Build history of the part. All positions in model axes, mm. A direction names the side the tool comes from. Coordinates: 2 decimals unless noted, no trailing zeros. Order: outer loops, then holes, each group sorted by start corner. A loop starts at its lowest first (then second) coordinate and runs counter-clockwise, first axis right, second up. Notation, with made-up numbers: M 41.25,18.5 L 74.25,18.5 A12 ccw 74.25,24.5 Z; hole C 88,-38 d11. An arc over 180 degrees is marked long. Use a Markdown table: item, result. Add a question column.
from build123d import *

# Parameters (mm, degrees)
SKETCH1_R                     = 8
BOSS_EXTRUDE1_DEPTH           = 1.6
SKETCH2_R                     = 6.07
BOSS_EXTRUDE2_DEPTH           = 8.2
BOSS_EXTRUDE3_START           = -1.6
SKETCH3_R                     = 8
BOSS_EXTRUDE3_DEPTH           = 1.6
SKETCH4_R                     = 6.35
BOSS_EXTRUDE4_DEPTH           = 5.6
F_5_0_5_DIAMETER_HOLE1_D      = 5
F_3_0_3_DIAMETER_HOLE1_REACH  = 23.882
F_3_0_3_DIAMETER_HOLE1_BORE_R = 1.5


with BuildPart() as part:
    # Sketch1 → Boss-Extrude1 (new body)
    with BuildSketch(Plane.XY.offset(1.6)):
        with Locations(Location((0, 0, 0), (0, 0, 180))):
            Circle(SKETCH1_R)
    extrude(amount=-BOSS_EXTRUDE1_DEPTH)

    # Sketch2 → Boss-Extrude2 (add)
    with BuildSketch(Plane.XY.offset(9.8)):
        with Locations(Location((0, 0, 0), (0, 0, 180))):
            Circle(SKETCH2_R)
    extrude(amount=-BOSS_EXTRUDE2_DEPTH)

    # Sketch3 → Boss-Extrude3 (add)
    with BuildSketch(Plane(origin=(0, 0, 9.8), x_dir=(-1, 0, 0), z_dir=(0, 0, -1)).offset(BOSS_EXTRUDE3_START)):
        Circle(SKETCH3_R)
    extrude(amount=BOSS_EXTRUDE3_DEPTH)

    # Sketch4 → Boss-Extrude4 (add)
    with BuildSketch(Plane.XY.offset(17)):
        Circle(SKETCH4_R)
    extrude(amount=-BOSS_EXTRUDE4_DEPTH)

    # Ø5.0 (5) Diameter Hole1 (through all)
    with Locations(Plane(origin=(0, 0, 0), x_dir=(-1, 0, 0), z_dir=(0, 0, -1))):
        with Locations((0, 0)):
            Hole(F_5_0_5_DIAMETER_HOLE1_D / 2)

    # Ø3.0 (3) Diameter Hole1 bore (on position points) → Ø3.0 (3) Diameter Hole1 (cut, up to next)
    with BuildSketch(Plane(origin=(-6.35, 0, 14.452836514), x_dir=(0, -1, 0), z_dir=(-1, 0, 0)), mode=Mode.PRIVATE) as f_3_0_3_diameter_hole1_sk1:
        Circle(F_3_0_3_DIAMETER_HOLE1_BORE_R)
    f_3_0_3_diameter_hole1_tool1 = extrude(f_3_0_3_diameter_hole1_sk1.sketch, amount=-F_3_0_3_DIAMETER_HOLE1_REACH, mode=Mode.PRIVATE) & part.part
    add(f_3_0_3_diameter_hole1_tool1.solids().sort_by_distance((-6.35, 0, 14.452837))[0], mode=Mode.SUBTRACT)


solid = part.part
(1) Drill centre lines: line 1 along Y through (x, z) = (0, 10.75); line 2 along Y through (x, z) = (0, 6.25); line 3 along Z through (x, y) = (-3.75, 5). Where is each one in solid material? Low to high. Write a range as from..to.
(2) Which spindle directions (+Z, -Z, +X, -X, +Y, -Y) get a long thin tool onto all of the face, cutting with end or side? Do faces 1 (the cylindrical face through (1.316, 5.926, 5.757)), 2 (the cylindrical face through (6.057, 1.907, 14.239)), 3 (the cylindrical face through (-4.2, 1.5, 14.5)), 4 (the cylindrical face through (1.73, -7.81, 10.61)). Say none if no direction does.
(3) Mould opens along Z. For faces 5 (the flat face through (-2, -2, 0)), 6 (the flat face through (3, 0, 17)), 7 (the flat face through (6, -2, 1.6)) say: released by +Z, released by -Z, zero draft, split by the parting line, or undercut.
(4) Slice it at D-D on z = 5.5. Give the cut face in (x, y).
(5) Slice it at C-C on x = -5.5. Give the cut face in (y, z), and give its area (3 significant figures).
(6) Drop flat-ended pins along their axis: P1, Ø3.5, axis at y = 0, z = 14.45, coming from the +X side; P2, Ø1, axis at y = -0.5, z = 4, coming from the +X side; P3, Ø4, axis at x = 0, y = 0, coming from the -Z side; P4, Ø3, axis at x = 5.5, z = 13.5, coming from the +Y side. Give the stop position or say it passes through.
(7) Slice it at B-B on y = 0. Give the cut face in (x, z).
(8) Slice it at A-A on x = 0. Give the cut face in (y, z), and give its area (3 significant figures).
Solutions:
| question | item | result |
|---|---|---|
| 1 | line 1 | -8..-2.5, 2.5..8 |
| 1 | line 2 | -6.07..-2.5, 2.5..6.07 |
| 1 | line 3 | 0..1.6, 9.8..17 |
| 2 | face 1 | none |
| 2 | face 2 | +Z |
| 2 | face 3 | -X |
| 2 | face 4 | +Z, -Z |
| 3 | face 5 | released by -Z |
| 3 | face 6 | released by +Z |
| 3 | face 7 | undercut |
| 4 | outline | C 0,0 d12.14; hole C 0,0 d5 |
| 5 | outline | M -5.81,0 L 5.81,0 L 5.81,1.6 L 2.57,1.6 L 2.57,9.8 L 5.81,9.8 L 5.81,11.4 L 3.17,11.4 L 3.17,17 L -3.17,17 L -3.17,11.4 L -5.81,11.4 L -5.81,9.8 L -2.57,9.8 L -2.57,1.6 L -5.81,1.6 Z; hole C 0,14.45 d3 |
| 5 | area | 108 mm² |
| 6 | P1 | x = 6.35 |
| 6 | P2 | x = 6.07 |
| 6 | P3 | through |
| 6 | P4 | y = 4.93 |
| 7 | outline | M -8,0 L -2.5,0 L -2.5,12.95 L -6.35,12.95 L -6.35,11.4 L -8,11.4 L -8,9.8 L -6.07,9.8 L -6.07,1.6 L -8,1.6 Z; M -6.35,15.95 L -2.5,15.95 L -2.5,17 L -6.35,17 Z; M 2.5,0 L 8,0 L 8,1.6 L 6.07,1.6 L 6.07,9.8 L 8,9.8 L 8,11.4 L 6.35,11.4 L 6.35,17 L 2.5,17 Z |
| 8 | outline | M -8,0 L -2.5,0 L -2.5,17 L -6.35,17 L -6.35,11.4 L -8,11.4 L -8,9.8 L -6.07,9.8 L -6.07,1.6 L -8,1.6 Z; M 2.5,0 L 8,0 L 8,1.6 L 6.07,1.6 L 6.07,9.8 L 8,9.8 L 8,11.4 L 6.35,11.4 L 6.35,17 L 2.5,17 Z |
| 8 | area | 137 mm² |
